Check sheet for the drawn part. Datum: minimum x, y, z corner. Units: mm. Coordinates: 2 decimals unless noted, no trailing zeros. Order: outer loops, then holes, each group sorted by start corner. A loop starts at its lowest first (then second) coordinate and runs counter-clockwise, first axis right, second up. Notation, with made-up numbers: (67, -0.5) - (79, -0.5) arc R18 ccw to (79, 28.5) - close; hole circle Ø9 at (66, -33). An arc over 180 degrees is marked (long way). Put each result on its own line as item: value.
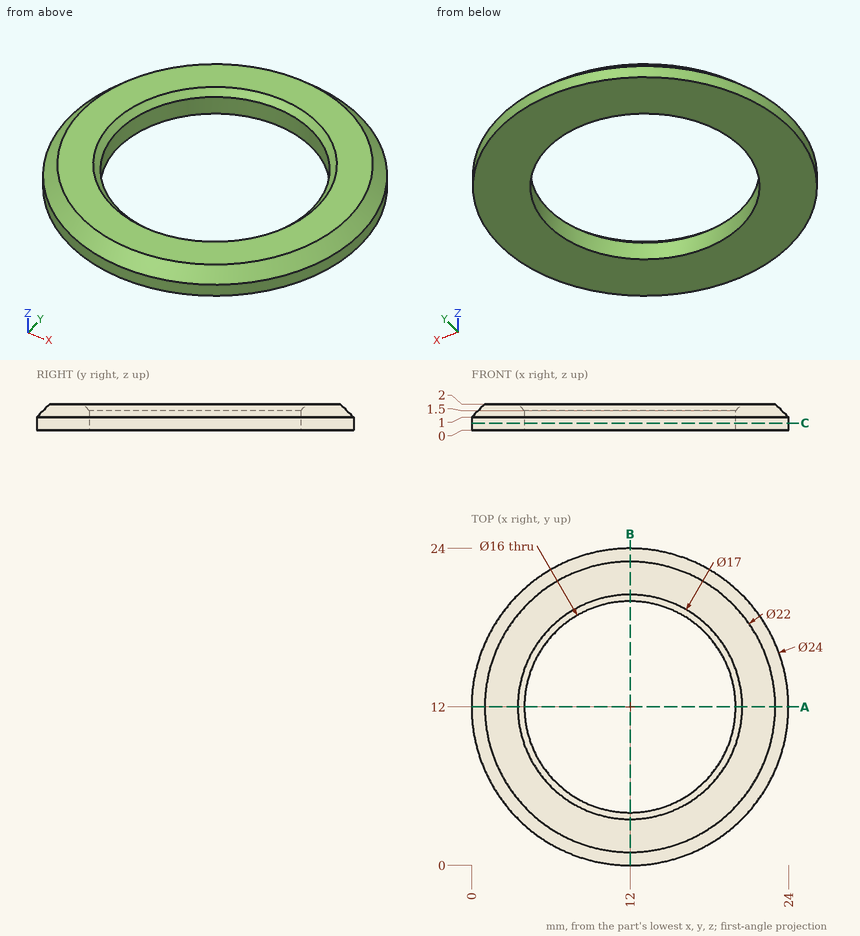
Q1. Depth check by flat-ended pin: pin 1 Ø3 at (x, y) = (18, 10.5) entering from +Z. Enter the tip coordinate at first touch or a pass-through.
Answer block:
pin 1: passes through
Q2. Section check C-C on z = 0.55. Record the boundary of the cut face in (x, y).
Answer block:
outline: circle Ø24 at (12, 12); hole circle Ø16 at (12, 12)
Q3. Thickness scan on L1, parallel to Y at x = 12, z = 0.75; L2, parallel to Y at x = 14.25, z = 1.25; L3, parallel to X at y = 16.5, z = 0.8. Record the ranges inside material, lowest first. Write a range as [from, to].
Answer block:
L1: y = [0, 4], [20, 24]
L2: y = [0.47, 4.32], [19.68, 23.53]
L3: x = [0.88, 5.39], [18.61, 23.12]
Q4. Section check A-A on y = 12. Record the boundary of the cut face in (x, z).
Answer block:
outline: (0, 0) - (4, 0) - (4, 1.5) - (3.5, 2) - (1, 2) - (0, 1) - close; (20, 0) - (24, 0) - (24, 1) - (23, 2) - (20.5, 2) - (20, 1.5) - close
